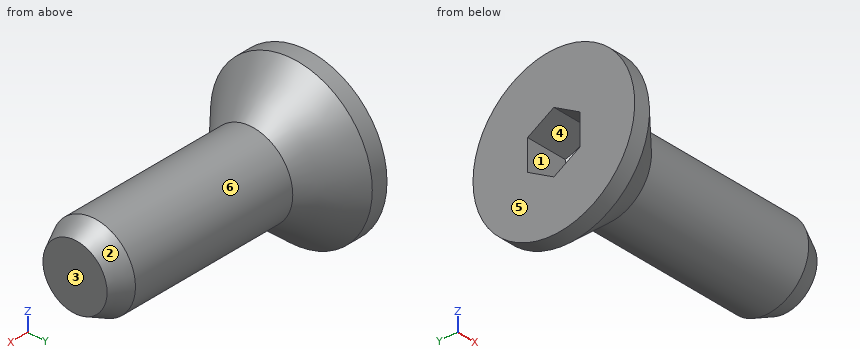
Autodesk Inventor part; units mm, degrees
ref_plane "Work Plane1" through (104.775, 0, 0) normal (0, 0, -1) x (1, 0, 0)
ref_plane "YZ Plane" through (0, 0, 0) normal (1, 0, 0) x (0, 1, 0)
ref_plane "XZ Plane" through (0, 0, 0) normal (0, 1, 0) x (-1, 0, 0)
sketch "Sketch1" plane through (0, 0, 0) normal (0, 0, 1) x (1, 0, 0)
  line L0 (9.525, 0) -> (9.525, 1.5875)
  line L1 (9.525, 1.5875) -> (3.8735, 1.5875)
  line L2 (3.8735, 1.5875) -> (2.286, 1.5875)
  line L3 (0, 3.048) -> (0, 1.1438)
  line L4 (0, 1.1438) -> (1.5494, 1.1438)
  line L5 (1.5494, 1.1438) -> (2.2098, 0)
  line L6 (2.2098, 0) -> (9.525, 0)
  line L7 (0, 3.048) -> (0.6059, 3.048)
  line L8 (0.6059, 3.048) -> (2.286, 1.5875)
  line L9 (2.286, 1.5875) -> (2.286, 1.5875)
  line L10 (3.8735, 1.5875) -> (2.286, 1.5875) construction
  line L11 (2.286, 1.5875) -> (2.286, 1.5875)
  line L12 (-1.905, 0) -> (11.43, 0)
  line L13 (0, -0.6096) -> (0, 3.6576)
  dimension "d0" = 9.525
  dimension "d1" = 5.6515
  dimension "d2" = 1.5494
  dimension "d3" = 3.175
  dimension "d6" = 2.286
  dimension "d7" = 41
  dimension "d8" = 2.2877
  dimension "d9" = 60
  dimension "d10" = 6.096
  dimension "d11" = 3.175
  dimension "d12" = 1.5875
revolve "Body" add sketch "Sketch1" angle 360 about axis through (2.2098, 0, 0) along (1, 0, 0) contours L6 L5 L4 L3 L7 L8 L2 L1 L0
sketch "Sketch2" plane through (0, 0, 0) normal (-1, 0, 0) x (0, 0, 1)
  circle A0 centre (0, 0) radius 1.1438
  line L0 (0, -4.2672) -> (0, 4.2672)
  line L1 (-4.2672, 0) -> (4.2672, 0)
  line L2 (1.1438, 0) -> (0.5719, -0.9906)
  line L3 (0.5719, -0.9906) -> (-0.5719, -0.9906)
  line L4 (-0.5719, -0.9906) -> (-1.1438, 0)
  line L5 (-1.1438, 0) -> (-0.5719, 0.9906)
  line L6 (-0.5719, 0.9906) -> (0.5719, 0.9906)
  line L7 (0.5719, 0.9906) -> (1.1438, 0)
  point P0 (0, 1.1438)
extrude "Slot" add sketch "Sketch2" against normal up to next contours L7 A0 | A0 L2 | L6 L0 A0 | A0 L0 L3 | L0 L6 A0 | A0 L3 L0 | L4 A0 | A0 L5
thread "Thread"
chamfer "Chamfer1" distance 0.3785 distance2 0.7569 1 edges at (9.525, -1.5875, 0) measured on face at (9.525, -0.1593, -0.6099)
ref_plane "Work Plane1" through (104.775, 0, 0) normal (0, 0, -1) x (1, 0, 0)
equation "\"d15\" = GEL"
equation "\"d17\" = -0.5 * SPD + 0.5 * GD"
equation "\"d18\" = GUL"
equation "\"d0\" = NLG"
equation "\"d1\" = GEL"
equation "\"d2\" = INTI"
equation "\"d3\" = GD"
equation "\"d6\" = KOH"
equation "\"d7\" = 0.5 * SEWI"
equation "\"d8\" = 1.1547 * SW"
equation "\"d10\" = KOD"
equation "\"d11\" = BDM"
equation "\"d12\" = GAL"
equation "\"NLG\" = 9.525"
equation "\"INTI\" = 1.5494"
equation "\"GEL\" = 5.6515"
equation "\"GAL\" = 1.5875"
equation "\"KOH\" = 2.286"
equation "\"KOD\" = 6.096"
equation "\"GUL\" = 0.75692"
equation "\"SPD\" = 2.41808"
equation "\"BDM\" = NND"
equation "\"GD\" = NND"
equation "\"SEWI\" = 82deg"
equation "\"SW\" = 1.9812"
equation "\"TOA\" = 30deg"
equation "\"GD1\" = SPD"
equation "\"THREADDIA\" = 3.175"
equation "\"HHPTC\" = 0.635"
equation "\"NND\" = 3.175"
equation "\"E0\" = 1.155 * SW"
properties part number "ANSI B18.3 - 5-40 UNC x 0.375, HSFCHCSI" material "Steel, Mild"
Verification items for the finished model (mm, model axes). Face numbers are marked on the shaded views. A direction names the side the tool comes from. Give positions to 0.01 mm unless a question says otherwise; leave off trailing zeros. Order: outer loops, then holes, each group sorted by start corner. A loop starts at its lowest first (then second) coordinate and runs counter-clockwise, first axis right, second up. Notation, with made-up numbers: (-25.75, -27.5) -> (-12.75, -27.5) arc R24 ccw to (-12.75, -2.5) -> close; hole circle Ø11 at (75, -26.5). An arc over 180 degrees is marked (long way). One line per item, written item: value.
(1) Draft check along Y on the marked faces 1, 2 and 3. Enter one of: pulls with the +Y half, pulls with the -Y half, needs draft (parallel to the pull), parting line crosses it, or undercut.
Final values:
face 1: undercut
face 2: parting line crosses it
face 3: needs draft
(2) Sectioned sample at B-B on x = 8. Record the cut outline in (y, z) (1 decimal), then the cut area to 3 significant figures.
Final values:
outline: circle Ø3.2 at (0, 0)
area: 7.92 mm^2
(3) Tool access check on the marked faces 4, 5 and 6. Record the directions out of +Z, -Z, +X, -X, +Y, -Y that give a thin tool (end or side, any length) a straight path to the whole face; none if there is none.
Final values:
face 4: -X
face 5: +Z, -Z, -X, +Y, -Y
face 6: +X
(4) Gauge pin test, flat ends, axial feed: pin 1 (1.5 mm diameter, centred on x = 7.5, y = 1.5, fed in from -Z); pin 2 (1.5 mm diameter, centred on x = 8, y = 2, fed in from +Z); pin 3 (1.5 mm diameter, centred on x = 8, z = -2, fed in from -Y). Record the tip position at first contact, or that the pin passes through.
Final values:
pin 1: z = -1.4
pin 2: z = 0.98
pin 3: y = -0.98
(5) Sectioned sample at A-A on x = 1. Record the cut outline in (y, z).
Final values:
outline: circle Ø5.41 at (0, 0); hole (-0.99, -0.57) -> (0, -1.14) -> (0.99, -0.57) -> (0.99, 0.57) -> (0, 1.14) -> (-0.99, 0.57) -> close
(6) Scan lines: line 1 along Z through (x, y) = (8.75, 0); line 2 along Y through (x, z) = (4, 1.25); line 3 along Z through (x, y) = (1.25, 2). Record each from-to range of solid material in increasing order. Write a range as [from, to].
Final values:
line 1: [-1.59, 1.59]
line 2: [-0.98, 0.98]
line 3: [-1.48, 1.48]
